Can you work these out from the model? Positions are in its coordinate system, mm. Give positions to 0.01 mm unless a question says otherwise; leave off trailing zeros. Loops run counter-clockwise (first coordinate to the right, second up) from the corner with the lowest first, then second, coordinate; pieces in that order, holes last. Notation, with made-up numbers: (89, 80.25) -> (137, 80.25) arc R17 cw to (137, 103.25) -> close; hole circle Ø2 at (71.25, 89.25). An arc over 180 degrees is marked (long way). One line per question, with ' | ' between items.
from build123d import *

# Parameters (mm, degrees)
F0_R     = 150
F0_R_2   = 13
F0_R_3   = 91.5
F1_DEPTH = 25


with BuildPart() as f1:
    # F0 (on Top) → F1 (new body)
    with BuildSketch(Plane.XY):
        with Locations((-15.279851, 11.636195)):
            Circle(F0_R)
        with Locations((-79.44674, -82.758747)):
            Circle(F0_R_2, mode=Mode.SUBTRACT)
        with Locations((-127.347842, -36.266502)):
            Circle(F0_R_2, mode=Mode.SUBTRACT)
        with Locations((2.266906, -95.438458)):
            Circle(F0_R_2, mode=Mode.SUBTRACT)
        with Locations((75.527415, -70.079044)):
            Circle(F0_R_2, mode=Mode.SUBTRACT)
        with Locations((90.320408, -1.045102)):
            Circle(F0_R_2, mode=Mode.SUBTRACT)
        with Locations((-135.09655, 44.742718)):
            Circle(F0_R_2, mode=Mode.SUBTRACT)
        with Locations((-95.648579, 109.550089)):
            Circle(F0_R_2, mode=Mode.SUBTRACT)
        with Locations((-15.279851, 11.636195)):
            Circle(F0_R_3, mode=Mode.SUBTRACT)
        with Locations((79.049557, 75.033121)):
            Circle(F0_R_2, mode=Mode.SUBTRACT)
        with Locations((41.010443, 119.412079)):
            Circle(F0_R_2, mode=Mode.SUBTRACT)
        with Locations((-13.23051, 131.387368)):
            Circle(F0_R_2, mode=Mode.SUBTRACT)
    extrude(amount=F1_DEPTH)


solid = f1.part
Q1. If we section it at B-B (y = -75.5): Write out the boundary of the cut face in (x, z), plus the area to 3 significant figures.
Entries:
outline: (-137.38, 0) -> (-90.23, 0) -> (-90.23, 25) -> (-137.38, 25) -> close; (-68.66, 0) -> (-43.2, 0) -> (-43.2, 25) -> (-68.66, 25) -> close; (12.64, 0) -> (63.71, 0) -> (63.71, 25) -> (12.64, 25) -> close; (87.34, 0) -> (106.82, 0) -> (106.82, 25) -> (87.34, 25) -> close | area: 3,580 mm²
Q2. For pin 1 Ø23.5 at (x, y) = (41.01, 119.41) entering from -Z; pin 2 Ø3 at (x, z) = (101, 15.5) entering from -Y; pin 3 Ø12 at (x, z) = (79.5, 6.5) entering from +Y; pin 4 Ø5 at (y, z) = (78, 3) entering from -X, each with a flat end and sliding along its axis, tell me the tip position at first contact or that it passes through.
Entries:
pin 1: through | pin 2: y = -84.93 | pin 3: y = 132.54 | pin 4: x = -151.01
Q3. If we section it at C-C (x = -53): Write out the boundary of the cut face in (y, z), plus the area to 3 significant figures.
Entries:
outline: (-133.54, 0) -> (-71.73, 0) -> (-71.73, 25) -> (-133.54, 25) -> close; (95, 0) -> (156.82, 0) -> (156.82, 25) -> (95, 25) -> close | area: 3,090 mm²
Q4. If I drill on probe 1 along Y at (x, z) = (-87, 2.5); probe 2 along Y at (x, z) = (-3.5, 14); probe 3 along Y at (x, z) = (12, 11.75), over which ranges is the centre line in solid material (lowest first)? Write a range as from..to.
Entries:
probe 1: -120.11..-93.34, -72.18..-45.18, 68.46..99.84, 119.26..143.38 | probe 2: -137.9..-107.09, -83.79..-79.1, 102.37..122.77, 140.01..161.17 | probe 3: -135.86..-104.06, -86.82..-75.7, 98.97..159.13
Q5. If we section it at D-D (z = 18.5): State how many separate pieces and enclosed holes the cut face has, plus the area to 3 significant figures.
Entries:
separate pieces: 1 | enclosed holes: 11 | area: 39,100 mm²
Q6. If we section it at A-A (x = -18.5): Write out the boundary of the cut face in (y, z).
Entries:
outline: (-138.33, 0) -> (-79.81, 0) -> (-79.81, 25) -> (-138.33, 25) -> close; (103.08, 0) -> (119.5, 0) -> (119.5, 25) -> (103.08, 25) -> close; (143.27, 0) -> (161.6, 0) -> (161.6, 25) -> (143.27, 25) -> close
Q7. If we mould it in two halves opening along X, with no side actions, what happens to faces 1 (the face through (-17, -86, 0)), 2 (the face through (-47.797, -134.797, 12.325)), 3 (the face through (-115.34, -41.25, 12.32))? For each: pulls with the +X half, pulls with the -X half, needs draft (parallel to the pull), parting line crosses it, or undercut.
Entries:
face 1: needs draft | face 2: parting line crosses it | face 3: undercut
